from build123d import *

# Parameters (mm, degrees)
PAD025_DEPTH    = 2
FILLET003_R     = 2.380952
SKETCH049_R     = 1.25
POCKET014_DEPTH = 2
SKETCH050_W     = 5
SKETCH050_H     = 10
PAD026_DEPTH    = 3
SKETCH051_R     = 1
PAD027_DEPTH    = 5


with BuildPart() as part:
    # Sketch048 → Pad025 (new body)
    with BuildSketch(Plane.XY):
        Polygon((-2.5, -2.5), (11.08, -2.5), (11.08, 2.5), (2.5, 2.5), (2.5, 12.5), (-2.5, 12.5), align=None)
    extrude(amount=PAD025_DEPTH)

    # Fillet003
    fillet003_edges = [part.edges().sort_by_distance(p)[0] for p in [
        (11.08, 2.5, 1),
        (11.08, -2.5, 1),
    ]]
    fillet(fillet003_edges, radius=FILLET003_R)

    # Sketch049 (on Face2 of Fillet003) → Pocket014 (cut)
    with BuildSketch(Plane(origin=(0, 0, 0), x_dir=(1, 0, 0), z_dir=(0, 0, -1))):
        Circle(SKETCH049_R)
        with Locations((8.58, 0)):
            Circle(SKETCH049_R)
    extrude(amount=-POCKET014_DEPTH, mode=Mode.SUBTRACT)

    # Sketch050 (on Face2 of Fillet003) → Pad026 (join)
    with BuildSketch(Plane(origin=(0, 0, 0), x_dir=(1, 0, 0), z_dir=(0, 0, -1))):
        with Locations((0, -7.5)):
            Rectangle(SKETCH050_W, SKETCH050_H)
    extrude(amount=PAD026_DEPTH)

    # Sketch051 (on Face12 of Pad026) → Pad027 (join)
    with BuildSketch(Plane(origin=(0, 12.5, 0), x_dir=(-1, 0, 0), z_dir=(0, 1, 0))):
        with Locations((0, -0.5)):
            Circle(SKETCH051_R)
    extrude(amount=PAD027_DEPTH)


with BuildPart() as part_1:
    # Body010 placement: moved
    add(part.part.moved(Location((119.92, 14.5, 6.25))))


solid = part_1.part
Geometry: final body of the model. Coordinates: model frame, mm. A direction names the side the tool comes from. Coordinates: 2 decimals unless noted, no trailing zeros. Order: outer loops, then holes, each group sorted by start corner. A loop starts at its lowest first (then second) coordinate and runs counter-clockwise, first axis right, second up.
(1) Draft query along X for faces 1 (the face through (121.11, 14.12, 7.24)), 2 (the face through (126, 17, 7)), 3 (the face through (117.42, 21, 6)). Return one class per face: pulls with the +X half, pulls with the -X half, needs draft (parallel to the pull), parting line crosses it, or undercut.
(2) Section query D-D (x = 129). Return the cut outline in (y, z), plus the area to 3 significant figures.
(3) First-contact query: pin 1 (1.5 mm diameter, centred on x = 128.5, y = 14.5, fed in from -Z); pin 2 (0.9 mm diameter, centred on x = 119.5, z = 5.5, fed in from -Y); pin 3 (0.6 mm diameter, centred on x = 125, z = 7, fed in from +Y); pin 4 (2.5 mm diameter, centred on y = 24.5, z = 4.5, fed in from +X). Flat tips, straight axial feed; report the tip coordinate or a pass-through.
(4) Section query B-B (z = 7.2). Return the cut outline in (x, y), plus the area to 3 significant figures.
(5) Section query C-C (z = 5.75). Return the cut outline in (x, y).
(6) Material intervals for probe 1 along X at (y, z) = (14.5, 7.7); probe 2 along Y at (x, z) = (119.92, 7.65); probe 3 along Y at (x, z) = (128.5, 7.8), sorted ascending.
(7) Access query for faces 4 (the face through (120, 27, 7)), 5 (the face through (123, 12, 7)), 6 (the face through (122.42, 22, 6)), 7 (the face through (124, 15, 6.25)). Directions: +Z, -Z, +X, -X, +Y, -Y. A direction counts if a zero-diameter tool reaches every point of the face in a straight line with its end or side. Return the directions, or none.
(8) Section query A-A (x = 127.5). Return the cut outline in (y, z), plus the area to 3 significant figures.
Solution:
1. face 1: undercut
1. face 2: needs draft
1. face 3: pulls with the -X half
2. outline: (12.03, 6.25) - (13.35, 6.25) - (13.35, 8.25) - (12.03, 8.25) - close; (15.65, 6.25) - (16.97, 6.25) - (16.97, 8.25) - (15.65, 8.25) - close
2. area: 5.29 mm2
3. pin 1: passes through
3. pin 2: stops at y = 17
3. pin 3: stops at y = 17
3. pin 4: stops at x = 122.42
4. outline: (117.42, 12) - (128.62, 12) arc R2.38 ccw to (131, 14.38) - (131, 14.62) arc R2.38 ccw to (128.62, 17) - (122.42, 17) - (122.42, 27) - (117.42, 27) - close; hole circle Ø2.5 at (119.92, 14.5); hole circle Ø2.5 at (128.5, 14.5)
4. area: 106 mm2
5. outline: (117.42, 17) - (122.42, 17) - (122.42, 27) - (120.92, 27) - (120.92, 32) - (118.92, 32) - (118.92, 27) - (117.42, 27) - close
6. probe 1: x = 117.42 to 118.67, 121.17 to 127.25, 129.75 to 131
6. probe 2: y = 12 to 13.25, 15.75 to 27
6. probe 3: y = 12 to 13.25, 15.75 to 17
7. face 4: +Y
7. face 5: +Z, -Z, +X, -X, -Y
7. face 6: +Z, -Z, +X, +Y
7. face 7: -Z, +X, -X, -Y
8. outline: (12, 6.25) - (13.75, 6.25) - (13.75, 8.25) - (12, 8.25) - close; (15.25, 6.25) - (17, 6.25) - (17, 8.25) - (15.25, 8.25) - close
8. area: 7.00 mm2
